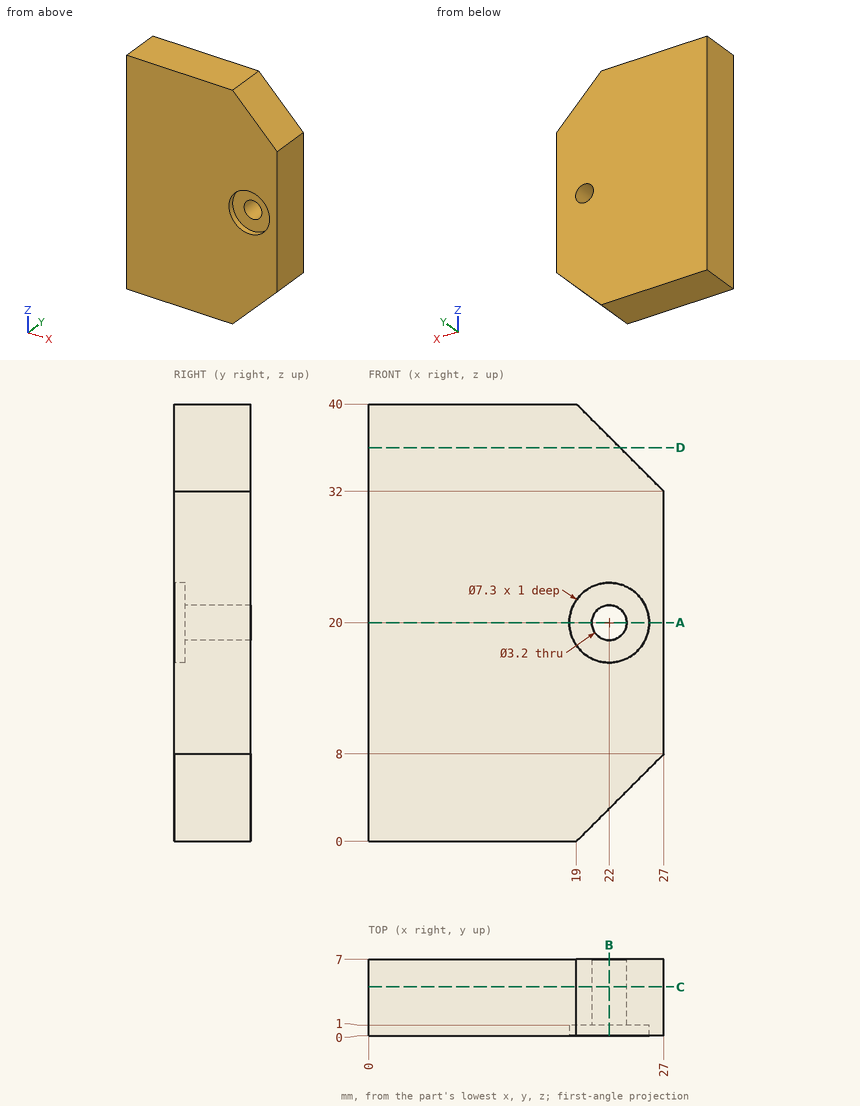
Study the drawing (mm; zero at the part's minimum x, y, z) and answer. Coordinates: 2 decimals unless noted, no trailing zeros. Loops run counter-clockwise (first coordinate to the right, second up) from the corner with the lowest first, then second, coordinate; pieces in that order, holes last. Notation, with made-up numbers: M -15,31 L 30,31 A21 ccw 30,52 Z; hole C -3,88.25 d5. An arc over 180 degrees is marked long. Answer as a JSON object with one key per item and string values. Group by question number.
Item 1: Section D-D (z = 36) is taken. Write down the section's boundary in (x, y).
Item 2: Consider L1, parallel to X at y = 5.45, z = 20; L2, parallel to X at y = 0.55, z = 20; L3, parallel to Z at x = 22, y = 2.2. Determine where each line is inside the solid, lowest interval first.
Item 3: Section B-B (x = 22) is taken. Write down the section's boundary in (y, z).
Item 4: Section A-A (z = 20) is taken. Write down the section's boundary in (x, y).
Item 5: Section C-C (y = 4.5) is taken. Write down the section's boundary in (x, z), and give its area (3 significant figures).
Solved:
{
 "1": {"outline": "M 0,0 L 23,0 L 23,7 L 0,7 Z"},
 "2": {"L1": "x = 0 to 20.4, 23.6 to 27", "L2": "x = 0 to 18.35, 25.65 to 27", "L3": "z = 3 to 18.4, 21.6 to 37"},
 "3": {"outline": "M 0,3 L 7,3 L 7,18.4 L 1,18.4 L 1,16.35 L 0,16.35 Z; M 0,23.65 L 1,23.65 L 1,21.6 L 7,21.6 L 7,37 L 0,37 Z"},
 "4": {"outline": "M 0,0 L 18.35,0 L 18.35,1 L 20.4,1 L 20.4,7 L 0,7 Z; M 23.6,1 L 25.65,1 L 25.65,0 L 27,0 L 27,7 L 23.6,7 Z"},
 "5": {"outline": "M 0,0 L 19,0 L 27,8 L 27,32 L 19,40 L 0,40 Z; hole C 22,20 d3.2", "area": "1,010 mm2"}
}
